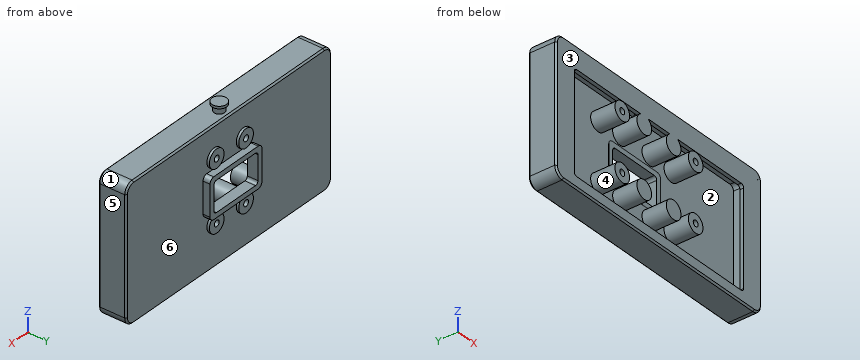
from build123d import *

# Parameters (mm, degrees)
BOSS_EXTRUDE1_START  = 50
BOSS_EXTRUDE1_DEPTH  = 9.2
CHAMFER1_SIZE        = 0.5
CHAMFER2_SIZE        = 0.5
BOSS_EXTRUDE2_START  = 49
BOSS_EXTRUDE2_DEPTH  = 9
BOSS_EXTRUDE3_START  = 50
SKETCH3_R            = 3
BOSS_EXTRUDE3_DEPTH  = 8.01
BOSS_EXTRUDE4_START  = 49
SKETCH4_R            = 1
BOSS_EXTRUDE4_DEPTH  = 9.4
BOSS_EXTRUDE5_START  = 50
SKETCH5_R            = 3
BOSS_EXTRUDE5_DEPTH  = 8.01
BOSS_EXTRUDE6_START  = 49
SKETCH6_R            = 1
BOSS_EXTRUDE6_DEPTH  = 9.4
BOSS_EXTRUDE7_START  = 50
SKETCH7_R            = 3
BOSS_EXTRUDE7_DEPTH  = 8.01
BOSS_EXTRUDE8_START  = 49
SKETCH8_R            = 1
BOSS_EXTRUDE8_DEPTH  = 9.4
BOSS_EXTRUDE9_START  = 50
SKETCH9_R            = 3
BOSS_EXTRUDE9_DEPTH  = 8.01
BOSS_EXTRUDE10_START = 49
SKETCH10_R           = 1
BOSS_EXTRUDE10_DEPTH = 9.4
BOSS_EXTRUDE11_START = 50
SKETCH11_R           = 3
BOSS_EXTRUDE11_DEPTH = 10
BOSS_EXTRUDE12_START = 51.5
SKETCH12_R           = 1
BOSS_EXTRUDE12_DEPTH = 9.5
BOSS_EXTRUDE13_START = 50
SKETCH13_R           = 3
BOSS_EXTRUDE13_DEPTH = 10
BOSS_EXTRUDE14_START = 51.5
SKETCH14_R           = 1
BOSS_EXTRUDE14_DEPTH = 9.5
BOSS_EXTRUDE15_START = 50
SKETCH15_R           = 3
BOSS_EXTRUDE15_DEPTH = 10
BOSS_EXTRUDE16_START = 51.5
SKETCH16_R           = 1
BOSS_EXTRUDE16_DEPTH = 9.5
BOSS_EXTRUDE17_START = 50
SKETCH17_R           = 3
BOSS_EXTRUDE17_DEPTH = 10
BOSS_EXTRUDE18_START = 51.5
SKETCH18_R           = 1
BOSS_EXTRUDE18_DEPTH = 9.5
BOSS_EXTRUDE19_START = 78.39
SKETCH19_R           = 1.7
BOSS_EXTRUDE19_DEPTH = 3.71
BOSS_EXTRUDE20_START = 82.1
SKETCH20_R           = 2.4
BOSS_EXTRUDE20_DEPTH = 0.8
BOSS_EXTRUDE21_START = 50
BOSS_EXTRUDE21_DEPTH = 1.2
BOSS_EXTRUDE22_START = 57.99
BOSS_EXTRUDE22_DEPTH = 3.51
BOSS_EXTRUDE23_START = 49
BOSS_EXTRUDE23_DEPTH = 13


with BuildPart() as part:
    # Sketch1 → Boss-Extrude1 (new body)
    with BuildSketch(Plane(origin=(0, 0, 0), x_dir=(1, 0, 0), z_dir=(0, 1, 0)).offset(BOSS_EXTRUDE1_START)):
        with BuildLine():
            Line((-39, -36), (39, -36))
            ThreePointArc((39, -36), (41.121320344, -36.878679656), (42, -39))
            Line((42, -39), (42, -77))
            ThreePointArc((42, -77), (41.121320344, -79.121320344), (39, -80))
            Line((39, -80), (-39, -80))
            ThreePointArc((-39, -80), (-41.121320344, -79.121320344), (-42, -77))
            Line((-42, -77), (-42, -39))
            ThreePointArc((-42, -39), (-41.121320344, -36.878679656), (-39, -36))
        make_face()
    extrude(amount=BOSS_EXTRUDE1_DEPTH)

    # Chamfer1
    chamfer1_edges = [part.edges().sort_by_distance(p)[0] for p in [
        (0, 50, 80),
        (-41.121320344, 50, 79.121320344),
        (-42, 50, 58),
        (-41.121320344, 50, 36.878679656),
        (0, 50, 36),
        (41.121320344, 50, 36.878679656),
        (42, 50, 58),
        (41.121320344, 50, 79.121320344),
    ]]
    chamfer(chamfer1_edges, length=CHAMFER1_SIZE)

    # Chamfer2
    chamfer2_edges = [part.edges().sort_by_distance(p)[0] for p in [
        (-41.121320344, 59.2, 79.121320344),
        (0, 59.2, 80),
        (41.121320344, 59.2, 79.121320344),
        (42, 59.2, 58),
        (41.121320344, 59.2, 36.878679656),
        (0, 59.2, 36),
        (-41.121320344, 59.2, 36.878679656),
        (-42, 59.2, 58),
    ]]
    chamfer(chamfer2_edges, length=CHAMFER2_SIZE)


with BuildPart() as body_2:
    # Sketch2 → Boss-Extrude2 (new body)
    with BuildSketch(Plane(origin=(0, 0, 0), x_dir=(1, 0, 0), z_dir=(0, 1, 0)).offset(BOSS_EXTRUDE2_START)):
        with BuildLine():
            Line((-39, -37.6), (39, -37.6))
            ThreePointArc((39, -37.6), (39.989949494, -38.010050506), (40.4, -39))
            Line((40.4, -39), (40.4, -77))
            ThreePointArc((40.4, -77), (39.989949494, -77.989949494), (39, -78.4))
            Line((39, -78.4), (-39, -78.4))
            ThreePointArc((-39, -78.4), (-39.989949494, -77.989949494), (-40.4, -77))
            Line((-40.4, -77), (-40.4, -39))
            ThreePointArc((-40.4, -39), (-39.989949494, -38.010050506), (-39, -37.6))
        make_face()
    extrude(amount=BOSS_EXTRUDE2_DEPTH)


with BuildPart() as part_1:
    add(part.part)

    # Combine1: cut body 2
    add(body_2.part, mode=Mode.SUBTRACT)

    # Sketch3 → Boss-Extrude3 (add)
    with BuildSketch(Plane(origin=(0, 0, 0), x_dir=(1, 0, 0), z_dir=(0, 1, 0)).offset(BOSS_EXTRUDE3_START)):
        with Locations(Location((-15, -50.5, 0), (0, 0, 90))):
            Circle(SKETCH3_R)
    extrude(amount=BOSS_EXTRUDE3_DEPTH)


with BuildPart() as body_2_2:
    # Sketch4 → Boss-Extrude4 (new body)
    with BuildSketch(Plane(origin=(0, 0, 0), x_dir=(1, 0, 0), z_dir=(0, 1, 0)).offset(BOSS_EXTRUDE4_START)):
        with Locations(Location((-15, -50.5, 0), (0, 0, 90))):
            Circle(SKETCH4_R)
    extrude(amount=BOSS_EXTRUDE4_DEPTH)


with BuildPart() as part_2:
    add(part_1.part)

    # Combine2: cut body 2 2
    add(body_2_2.part, mode=Mode.SUBTRACT)

    # Sketch5 → Boss-Extrude5 (add)
    with BuildSketch(Plane(origin=(0, 0, 0), x_dir=(1, 0, 0), z_dir=(0, 1, 0)).offset(BOSS_EXTRUDE5_START)):
        with Locations(Location((-15, -69.5, 0), (0, 0, 90))):
            Circle(SKETCH5_R)
    extrude(amount=BOSS_EXTRUDE5_DEPTH)


with BuildPart() as body_2_3:
    # Sketch6 → Boss-Extrude6 (new body)
    with BuildSketch(Plane(origin=(0, 0, 0), x_dir=(1, 0, 0), z_dir=(0, 1, 0)).offset(BOSS_EXTRUDE6_START)):
        with Locations(Location((-15, -69.5, 0), (0, 0, 90))):
            Circle(SKETCH6_R)
    extrude(amount=BOSS_EXTRUDE6_DEPTH)


with BuildPart() as part_3:
    add(part_2.part)

    # Combine3: cut body 2 3
    add(body_2_3.part, mode=Mode.SUBTRACT)

    # Sketch7 → Boss-Extrude7 (add)
    with BuildSketch(Plane(origin=(0, 0, 0), x_dir=(1, 0, 0), z_dir=(0, 1, 0)).offset(BOSS_EXTRUDE7_START)):
        with Locations(Location((15, -50.5, 0), (0, 0, 90))):
            Circle(SKETCH7_R)
    extrude(amount=BOSS_EXTRUDE7_DEPTH)


with BuildPart() as body_2_4:
    # Sketch8 → Boss-Extrude8 (new body)
    with BuildSketch(Plane(origin=(0, 0, 0), x_dir=(1, 0, 0), z_dir=(0, 1, 0)).offset(BOSS_EXTRUDE8_START)):
        with Locations(Location((15, -50.5, 0), (0, 0, 90))):
            Circle(SKETCH8_R)
    extrude(amount=BOSS_EXTRUDE8_DEPTH)


with BuildPart() as part_4:
    add(part_3.part)

    # Combine4: cut body 2 4
    add(body_2_4.part, mode=Mode.SUBTRACT)

    # Sketch9 → Boss-Extrude9 (add)
    with BuildSketch(Plane(origin=(0, 0, 0), x_dir=(1, 0, 0), z_dir=(0, 1, 0)).offset(BOSS_EXTRUDE9_START)):
        with Locations(Location((15, -69.5, 0), (0, 0, 90))):
            Circle(SKETCH9_R)
    extrude(amount=BOSS_EXTRUDE9_DEPTH)


with BuildPart() as body_2_5:
    # Sketch10 → Boss-Extrude10 (new body)
    with BuildSketch(Plane(origin=(0, 0, 0), x_dir=(1, 0, 0), z_dir=(0, 1, 0)).offset(BOSS_EXTRUDE10_START)):
        with Locations(Location((15, -69.5, 0), (0, 0, 90))):
            Circle(SKETCH10_R)
    extrude(amount=BOSS_EXTRUDE10_DEPTH)


with BuildPart() as part_5:
    add(part_4.part)

    # Combine5: cut body 2 5
    add(body_2_5.part, mode=Mode.SUBTRACT)

    # Sketch11 → Boss-Extrude11 (add)
    with BuildSketch(Plane(origin=(0, 0, 0), x_dir=(1, 0, 0), z_dir=(0, 1, 0)).offset(BOSS_EXTRUDE11_START)):
        with Locations(Location((-6, -50, 0), (0, 0, 90))):
            Circle(SKETCH11_R)
    extrude(amount=BOSS_EXTRUDE11_DEPTH)


with BuildPart() as body_2_6:
    # Sketch12 → Boss-Extrude12 (new body)
    with BuildSketch(Plane(origin=(0, 0, 0), x_dir=(1, 0, 0), z_dir=(0, 1, 0)).offset(BOSS_EXTRUDE12_START)):
        with Locations(Location((-6, -50, 0), (0, 0, 270))):
            Circle(SKETCH12_R)
    extrude(amount=BOSS_EXTRUDE12_DEPTH)


with BuildPart() as part_6:
    add(part_5.part)

    # Combine6: cut body 2 6
    add(body_2_6.part, mode=Mode.SUBTRACT)

    # Sketch13 → Boss-Extrude13 (add)
    with BuildSketch(Plane(origin=(0, 0, 0), x_dir=(1, 0, 0), z_dir=(0, 1, 0)).offset(BOSS_EXTRUDE13_START)):
        with Locations(Location((-6, -70, 0), (0, 0, 90))):
            Circle(SKETCH13_R)
    extrude(amount=BOSS_EXTRUDE13_DEPTH)


with BuildPart() as body_2_7:
    # Sketch14 → Boss-Extrude14 (new body)
    with BuildSketch(Plane(origin=(0, 0, 0), x_dir=(1, 0, 0), z_dir=(0, 1, 0)).offset(BOSS_EXTRUDE14_START)):
        with Locations(Location((-6, -70, 0), (0, 0, 270))):
            Circle(SKETCH14_R)
    extrude(amount=BOSS_EXTRUDE14_DEPTH)


with BuildPart() as part_7:
    add(part_6.part)

    # Combine7: cut body 2 7
    add(body_2_7.part, mode=Mode.SUBTRACT)

    # Sketch15 → Boss-Extrude15 (add)
    with BuildSketch(Plane(origin=(0, 0, 0), x_dir=(1, 0, 0), z_dir=(0, 1, 0)).offset(BOSS_EXTRUDE15_START)):
        with Locations(Location((6, -50, 0), (0, 0, 90))):
            Circle(SKETCH15_R)
    extrude(amount=BOSS_EXTRUDE15_DEPTH)


with BuildPart() as body_2_8:
    # Sketch16 → Boss-Extrude16 (new body)
    with BuildSketch(Plane(origin=(0, 0, 0), x_dir=(1, 0, 0), z_dir=(0, 1, 0)).offset(BOSS_EXTRUDE16_START)):
        with Locations(Location((6, -50, 0), (0, 0, 270))):
            Circle(SKETCH16_R)
    extrude(amount=BOSS_EXTRUDE16_DEPTH)


with BuildPart() as part_8:
    add(part_7.part)

    # Combine8: cut body 2 8
    add(body_2_8.part, mode=Mode.SUBTRACT)

    # Sketch17 → Boss-Extrude17 (add)
    with BuildSketch(Plane(origin=(0, 0, 0), x_dir=(1, 0, 0), z_dir=(0, 1, 0)).offset(BOSS_EXTRUDE17_START)):
        with Locations(Location((6, -70, 0), (0, 0, 90))):
            Circle(SKETCH17_R)
    extrude(amount=BOSS_EXTRUDE17_DEPTH)


with BuildPart() as body_2_9:
    # Sketch18 → Boss-Extrude18 (new body)
    with BuildSketch(Plane(origin=(0, 0, 0), x_dir=(1, 0, 0), z_dir=(0, 1, 0)).offset(BOSS_EXTRUDE18_START)):
        with Locations(Location((6, -70, 0), (0, 0, 270))):
            Circle(SKETCH18_R)
    extrude(amount=BOSS_EXTRUDE18_DEPTH)


with BuildPart() as part_9:
    add(part_8.part)

    # Combine9: cut body 2 9
    add(body_2_9.part, mode=Mode.SUBTRACT)

    # Sketch19 → Boss-Extrude19 (add)
    with BuildSketch(Plane.XY.offset(BOSS_EXTRUDE19_START)):
        with Locations(Location((0, 56, 0), (0, 0, 180))):
            Circle(SKETCH19_R)
    extrude(amount=BOSS_EXTRUDE19_DEPTH)

    # Sketch20 → Boss-Extrude20 (add)
    with BuildSketch(Plane.XY.offset(BOSS_EXTRUDE20_START)):
        with Locations((0, 56)):
            Circle(SKETCH20_R)
    extrude(amount=BOSS_EXTRUDE20_DEPTH)

    # Sketch21 → Boss-Extrude21 (add)
    with BuildSketch(Plane(origin=(0, 0, 0), x_dir=(1, 0, 0), z_dir=(0, 1, 0)).offset(BOSS_EXTRUDE21_START)):
        with BuildLine():
            Line((-38.99, -37.59), (38.99, -37.59))
            ThreePointArc((38.99, -37.59), (39.979949494, -38.000050506), (40.39, -38.99))
            Line((40.39, -38.99), (40.39, -77.01))
            ThreePointArc((40.39, -77.01), (39.979949494, -77.999949494), (38.99, -78.41))
            Line((38.99, -78.41), (-38.99, -78.41))
            ThreePointArc((-38.99, -78.41), (-39.979949494, -77.999949494), (-40.39, -77.01))
            Line((-40.39, -77.01), (-40.39, -38.99))
            ThreePointArc((-40.39, -38.99), (-39.979949494, -38.000050506), (-38.99, -37.59))
        make_face()
        with BuildLine():
            Line((-33.6, -39.6), (33.6, -39.6))
            ThreePointArc((33.6, -39.6), (34.307106781, -39.892893219), (34.6, -40.6))
            Line((34.6, -40.6), (34.6, -71.6))
            ThreePointArc((34.6, -71.6), (34.307106781, -72.307106781), (33.6, -72.6))
            Line((33.6, -72.6), (-33.6, -72.6))
            ThreePointArc((-33.6, -72.6), (-34.307106781, -72.307106781), (-34.6, -71.6))
            Line((-34.6, -71.6), (-34.6, -40.6))
            ThreePointArc((-34.6, -40.6), (-34.307106781, -39.892893219), (-33.6, -39.6))
        make_face(mode=Mode.SUBTRACT)
    extrude(amount=BOSS_EXTRUDE21_DEPTH)

    # Sketch22 → Boss-Extrude22 (add)
    with BuildSketch(Plane(origin=(0, 0, 0), x_dir=(1, 0, 0), z_dir=(0, 1, 0)).offset(BOSS_EXTRUDE22_START)):
        with BuildLine():
            Line((-9.1, -53.4), (9.1, -53.4))
            ThreePointArc((9.1, -53.4), (10.160660172, -53.839339828), (10.6, -54.9))
            Line((10.6, -54.9), (10.6, -65.1))
            ThreePointArc((10.6, -65.1), (10.160660172, -66.160660172), (9.1, -66.6))
            Line((9.1, -66.6), (-9.1, -66.6))
            ThreePointArc((-9.1, -66.6), (-10.160660172, -66.160660172), (-10.6, -65.1))
            Line((-10.6, -65.1), (-10.6, -54.9))
            ThreePointArc((-10.6, -54.9), (-10.160660172, -53.839339828), (-9.1, -53.4))
        make_face()
    extrude(amount=BOSS_EXTRUDE22_DEPTH)


with BuildPart() as body_2_10:
    # Sketch23 → Boss-Extrude23 (new body)
    with BuildSketch(Plane(origin=(0, 0, 0), x_dir=(1, 0, 0), z_dir=(0, 1, 0)).offset(BOSS_EXTRUDE23_START)):
        with BuildLine():
            Line((-8, -55), (8, -55))
            ThreePointArc((8, -55), (8.707106781, -55.292893219), (9, -56))
            Line((9, -56), (9, -64))
            ThreePointArc((9, -64), (8.707106781, -64.707106781), (8, -65))
            Line((8, -65), (-8, -65))
            ThreePointArc((-8, -65), (-8.707106781, -64.707106781), (-9, -64))
            Line((-9, -64), (-9, -56))
            ThreePointArc((-9, -56), (-8.707106781, -55.292893219), (-8, -55))
        make_face()
    extrude(amount=BOSS_EXTRUDE23_DEPTH)


with BuildPart() as part_10:
    add(part_9.part)

    # Combine10: cut body 2 10
    add(body_2_10.part, mode=Mode.SUBTRACT)


solid = part_10.part
Here's how the part is built. I have some questions about the finished solid (model axes, mm). Face numbers are marked on the shaded views. A direction names the side the tool comes from. Give positions to 0.01 mm unless a question says otherwise; leave off trailing zeros. One line per item, written item: value.
Q1. If I drill on line 1 along Z through (x, y) = (-6, 58.25); line 2 along Y through (x, z) = (37, 60); line 3 along X through (y, z) = (57.5, 45.5), over which ranges is the centre line in solid material (lowest first)?
Answers follow:
line 1: 36 to 49, 51 to 55, 65 to 69, 71 to 80
line 2: 50 to 51.2, 58 to 59.2
line 3: -42 to -40.4, 40.4 to 42
Q2. Suppose I cut it at A-A on y = 56. State how many separate pieces and enclosed holes the cut face has, then the cut area to 3 significant figures.
Answers follow:
separate pieces: 9
enclosed holes: 9
area: 605 mm^2
Q3. We'd pull the mould along Y, two halves only. Please class the marked faces 1, 2 and 3: pulls with the +Y half, pulls with the -Y half, needs draft (parallel to the pull), parting line crosses it, or undercut.
Answers follow:
face 1: needs draft
face 2: undercut
face 3: pulls with the -Y half
Q4. On a 3-axis mill with a long thin cutter (end or side, diameter ignored), from which of +Z, -Z, +X, -X, +Y, -Y can I reach the whole of each face in a straight line? I mean the marked faces 4, 5 and 6. Say none if no direction works.
Answers follow:
face 4: -Y
face 5: +Z, -Z, +X, +Y, -Y
face 6: +Y
Q5. I'm going to push flat-ended pins straight in: pin 1 Ø5 at (x, y) = (-32, 51.5) entering from +Z; pin 2 Ø6.5 at (x, z) = (-1, 61) entering from -Y; pin 3 Ø2.5 at (x, z) = (6, 50) entering from +Y; pin 4 Ø0.6 at (x, z) = (-15, 70) entering from -Y. Where does each tip first touch, or does it pass through?
Answers follow:
pin 1: z = 80
pin 2: through
pin 3: y = 60
pin 4: y = 58.4
